Geometry check sheet. Reference: the model listing, model coordinates, mm. A direction names the side the tool comes from. Coordinates: 2 decimals unless noted, no trailing zeros. Loops run counter-clockwise (first coordinate to the right, second up) from the corner with the lowest first, then second, coordinate; pieces in that order, holes last.
from build123d import *

# Parameters (mm, degrees)
F0_R     = 1.5875
F0_R_2   = 1.8288
F1_DEPTH = 1.5875


with BuildPart() as f1:
    # F0 (on Top) → F1 (new body)
    with BuildSketch(Plane.XY):
        with BuildLine():
            ThreePointArc((28.575, -4.7625), (33.3375, 0), (28.575, 4.7625))
            Line((28.575, 4.7625), (-28.575, 4.7625))
            ThreePointArc((-28.575, 4.7625), (-33.3375, 0), (-28.575, -4.7625))
            Line((-28.575, -4.7625), (28.575, -4.7625))
        make_face()
        with Locations((-28.575, 0)):
            Circle(F0_R, mode=Mode.SUBTRACT)
        with Locations((-9.525, 0)):
            Circle(F0_R_2, mode=Mode.SUBTRACT)
        with BuildLine():
            ThreePointArc((3.175, 1.5875), (4.7625, 0), (3.175, -1.5875))
            Line((3.175, -1.5875), (-3.175, -1.5875))
            ThreePointArc((-3.175, -1.5875), (-4.7625, 0), (-3.175, 1.5875))
            Line((-3.175, 1.5875), (3.175, 1.5875))
        make_face(mode=Mode.SUBTRACT)
        with Locations((9.525, 0)):
            Circle(F0_R_2, mode=Mode.SUBTRACT)
        with Locations((28.575, 0)):
            Circle(F0_R, mode=Mode.SUBTRACT)
    extrude(amount=F1_DEPTH)


solid = f1.part
(1) Sectioned sample at C-C on x = -28. Record the cut outline in (y, z).
Findings:
outline: (-4.76, 0) - (-1.48, 0) - (-1.48, 1.59) - (-4.76, 1.59) - close; (1.48, 0) - (4.76, 0) - (4.76, 1.59) - (1.48, 1.59) - close
(2) Sectioned sample at B-B on z = 0.85. Record the cut outline in (x, y) (1 decimal).
Findings:
outline: (-28.6, -4.8) - (28.6, -4.8) arc R4.8 ccw to (28.6, 4.8) - (-28.6, 4.8) arc R4.8 ccw to start; hole circle Ø3.2 at (-28.6, 0); hole circle Ø3.7 at (-9.5, 0); hole (-3.2, -1.6) - (3.2, -1.6) arc R1.6 ccw to (3.2, 1.6) - (-3.2, 1.6) arc R1.6 ccw to start; hole circle Ø3.7 at (9.5, 0); hole circle Ø3.2 at (28.6, 0)
(3) Sectioned sample at A-A on y = 0. Record the cut outline in (x, z), and give its area (3 significant figures).
Findings:
outline: (-33.34, 0) - (-30.16, 0) - (-30.16, 1.59) - (-33.34, 1.59) - close; (-26.99, 0) - (-11.35, 0) - (-11.35, 1.59) - (-26.99, 1.59) - close; (-7.7, 0) - (-4.76, 0) - (-4.76, 1.59) - (-7.7, 1.59) - close; (4.76, 0) - (7.7, 0) - (7.7, 1.59) - (4.76, 1.59) - close; (11.35, 0) - (26.99, 0) - (26.99, 1.59) - (11.35, 1.59) - close; (30.16, 0) - (33.34, 0) - (33.34, 1.59) - (30.16, 1.59) - close
area: 69.0 mm2
(4) Access from +Z, -Z, +X, -X, +Y, -Y to the whole of each face (thin tool, end or side, straight path). Record for faces 5 (the cylindrical face through (33.336, -0.105, 0.783)), 6 (the cylindrical face through (4.762, 0.035, 0.783)).
Findings:
face 5: +Z, -Z, +X
face 6: +Z, -Z
(5) Scan lines: L1, parallel to X at y = -0.5, z = 0.4; L2, parallel to Y at x = -29.5, z = 0.8; L3, parallel to X at y = -0.25, z = 0.75. Record each from-to range of solid material in increasing order.
Findings:
L1: x = -33.31 to -30.08, -27.07 to -11.28, -7.77 to -4.68, 4.68 to 7.77, 11.28 to 27.07, 30.08 to 33.31
L2: y = -4.67 to -1.29, 1.29 to 4.67
L3: x = -33.33 to -30.14, -27.01 to -11.34, -7.71 to -4.74, 4.74 to 7.71, 11.34 to 27.01, 30.14 to 33.33
(6) Draft check along Y on faces 1 (the flat face through (0, -1.588, 1)), 2 (the cylindrical face through (-7.78, 0.55, 0.78)), 3 (the flat face through (0, 2, 0)), 4 (the flat face through (0, -4.762, 1)). Enter one of: +Y half, -Y half, draft (parallel to the pull), parting line (faces both ways), or undercut.
Findings:
face 1: undercut
face 2: undercut
face 3: draft
face 4: -Y half
